Print and shaded views of the part. All mm, measured from the part's lowest x, y and z. A direction names the side the tool comes from. Round coordinates to 2 decimals unless told otherwise and drop trailing zeros. Loops run counter-clockwise (first coordinate to the right, second up) from the corner with the lowest first, then second, coordinate; pieces in that order, holes last. Notation, with made-up numbers: (40, -6.75) - (94, -6.75) arc R28 ccw to (94, 12.25) - close; hole circle Ø11 at (17.5, 2.5). An arc over 180 degrees is marked (long way). Use one line per item in the form item = value.
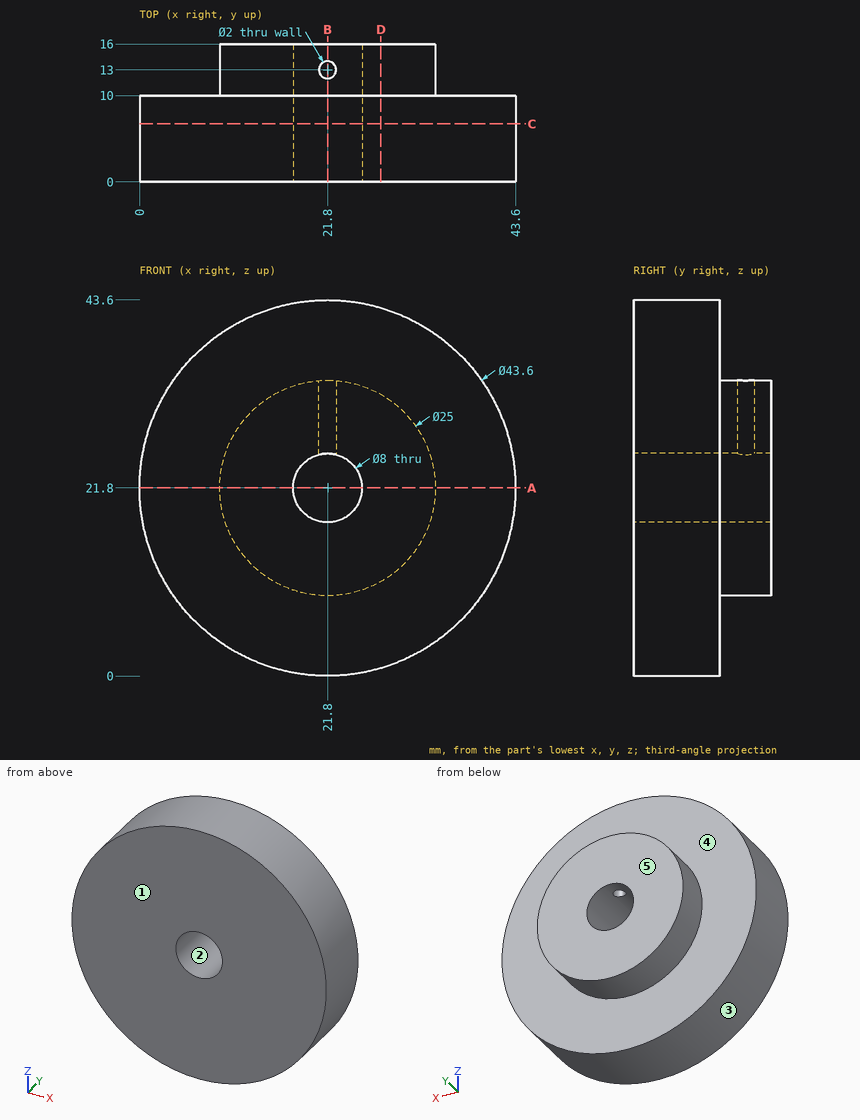
1) Slice it at D-D (x = 28). Write the cut outline in (y, z).
Report:
outline = (0, 0.9) - (10, 0.9) - (10, 10.95) - (16, 10.95) - (16, 32.65) - (10, 32.65) - (10, 42.7) - (0, 42.7) - close
2) Drill centre lines: probe 1 along Z at (x, y) = (22, 4) (3 decimals); probe 2 along X at (y, z) = (4.5, 21.8); probe 3 along Z at (x, y) = (23, 10.75). Where is each one in solid material? Low to high.
Report:
probe_1 = 0.001 to 17.805, 25.795 to 43.599
probe_2 = 0 to 17.8, 25.8 to 43.6
probe_3 = 9.36 to 17.98, 25.62 to 34.24
3) Slice it at B-B (x = 21.8). Write the cut outline in (y, z), plus the area to 3 significant figures.
Report:
outline = (0, 0) - (10, 0) - (10, 9.3) - (16, 9.3) - (16, 17.8) - (0, 17.8) - close; (0, 25.8) - (12, 25.8) - (12, 34.3) - (10, 34.3) - (10, 43.6) - (0, 43.6) - close; (14, 25.8) - (16, 25.8) - (16, 34.3) - (14, 34.3) - close
area = 441 mm^2
4) Slice it at A-A (z = 21.8). Write the cut outline in (x, y), plus the area to 3 significant figures.
Report:
outline = (0, 0) - (17.8, 0) - (17.8, 16) - (9.3, 16) - (9.3, 10) - (0, 10) - close; (25.8, 0) - (43.6, 0) - (43.6, 10) - (34.3, 10) - (34.3, 16) - (25.8, 16) - close
area = 458 mm^2
5) Flat gauge pins, fed straight in: pin 1 (3 mm diameter, centred on x = 29.5, y = 12, fed in from +Z); pin 2 (1.5 mm diameter, centred on x = 5.5, z = 10.5, fed in from +Y); pin 3 (6.5 mm diameter, centred on x = 21.8, z = 21.8, fed in from +Y); pin 4 (2 mm diameter, centred on y = 4.5, z = 33.5, fed in from -X). Where does each tip first touch, or does it go through?
Report:
pin_1 = 32.65
pin_2 = 10
pin_3 = through
pin_4 = 2.81
6) Tool access for the marked faces 4 and 5: list every direction of +Z, -Z, +X, -X, +Y, -Y with a clear straight run to the whole face (end or side of a thin tool).
Report:
face_4 = +Y
face_5 = +Z, -Z, +X, -X, +Y
7) Two-plate mould, pull along Z, no slides. Class the marked faces 1, 2 and 3: +Z half, -Z half, draft (parallel to the pull), parting line (faces both ways), or undercut.
Report:
face_1 = draft
face_2 = undercut
face_3 = parting line
8) Slice it at C-C (y = 6.75). Write the cut outline in (x, z), plus the area to 3 significant figures.
Report:
outline = circle Ø43.6 at (21.8, 21.8); hole circle Ø8 at (21.8, 21.8)
area = 1,440 mm^2
